Geometry check sheet. Reference: drawing and pictorial views, mm from the part's lowest x, y, z. A direction names the side the tool comes from. Give positions to 0.01 mm unless a question says otherwise; leave off trailing zeros. Loops run counter-clockwise (first coordinate to the right, second up) from the corner with the lowest first, then second, coordinate; pieces in that order, holes last. Notation, with made-up numbers: (-0.5, 3) - (19.5, 3) arc R24 cw to (19.5, 20) - close; hole circle Ø5 at (76.5, 59.5). An arc over 180 degrees is marked (long way). Use CSV: the item, a comma, the result in double quotes.
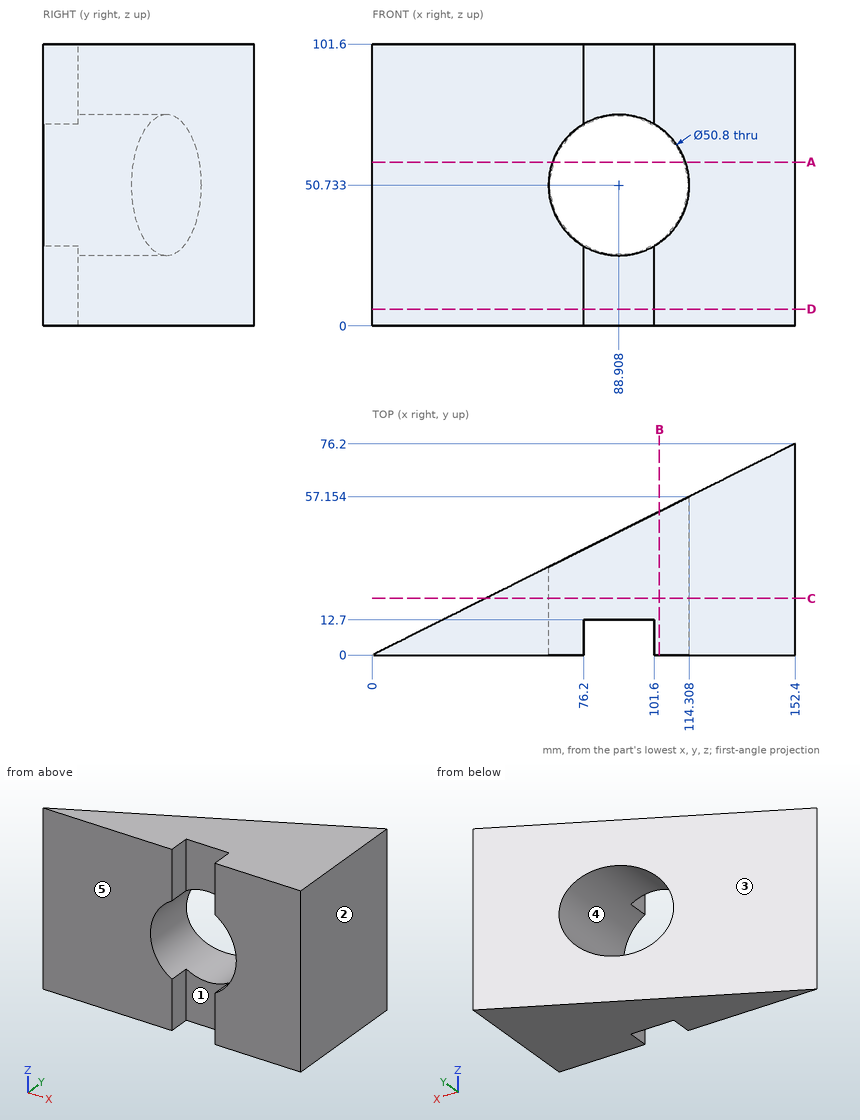
1. Sectioned sample at A-A, the plane z = 59. Record the boundary of the cut face in (x, y) (1 decimal), and give its area (3 significant figures).
Completed:
outline,"(0, 0) - (64.9, 0) - (64.9, 32.4) - close; (112.9, 0) - (152.4, 0) - (152.4, 76.2) - (112.9, 56.5) - close"
area,"3,670 mm²"
2. Release check for a two-part mould opening along X. For the marked faces 3, 4 and 5 record: released by +X, released by -X, zero draft, split by the parting line, or undercut.
Completed:
face 3,"released by -X"
face 4,"undercut"
face 5,"zero draft"
3. Sectioned sample at B-B, the plane x = 103.5. Record the boundary of the cut face in (y, z).
Completed:
outline,"(0, 0) - (51.75, 0) - (51.75, 29.94) - (0, 29.94) - close; (0, 71.52) - (51.75, 71.52) - (51.75, 101.6) - (0, 101.6) - close"
4. Sectioned sample at C-C, the plane y = 20.5. Record the boundary of the cut face in (x, z).
Completed:
outline,"(41, 0) - (152.4, 0) - (152.4, 101.6) - (41, 101.6) - close; hole circle Ø50.8 at (88.91, 50.73)"
5. Scan lines: line 1 along Z through (x, y) = (103, 31) (1 decimal); line 2 along Z through (x, y) = (79, 34) (1 decimal); line 3 along X through (y, z) = (20, 47) (1 decimal). Record each from-to range of solid material in increasing order.
Completed:
line 1,"z = 0 to 29.6, 71.9 to 101.6"
line 2,"z = 0 to 27.3, 74.1 to 101.6"
line 3,"x = 40 to 63.8, 114 to 152.4"
6. Go/stop test with flat-tipped pins: pin 1 Ø20.5 at (x, z) = (88.5, 84) entering from -Y; pin 2 Ø4 at (y, z) = (6, 14) entering from -X; pin 3 Ø10 at (x, z) = (106, 32.5) entering from -Y; pin 4 Ø2 at (y, z) = (32, 55) entering from -X. Record where each tip stops, or that it passes through.
Completed:
pin 1,"stops at y = 12.7"
pin 2,"stops at x = 8"
pin 3,"stops at y = 0"
pin 4,"stops at x = 62"
7. Sectioned sample at D-D, the plane z = 6. Record the boundary of the cut face in (x, y), and give its area (3 significant figures).
Completed:
outline,"(0, 0) - (76.2, 0) - (76.2, 12.7) - (101.6, 12.7) - (101.6, 0) - (152.4, 0) - (152.4, 76.2) - close"
area,"5,480 mm²"
8. Set-up check for the marked faces 1 and 2: record each of +Z, -Z, +X, -X, +Y, -Y from which the full face is reachable in a straight line by a thin tool's end or side.
Completed:
face 1,"+Z, -Z, -Y"
face 2,"+Z, -Z, +X, +Y, -Y"
